Design review of the part built by this model. Coordinates are the model's own, in mm. Face numbers are marked on the shaded views. A direction names the side the tool comes from. Give positions to 0.01 mm unless a question says otherwise; leave off trailing zeros. Write each loop counter-clockwise with the first axis right and the second up, starting at its lowest first coordinate (ties: lowest second). Pieces come first, ordered by that corner, then holes. Notation, with made-up numbers: (21, 75.25) -> (59, 75.25) arc R17 ccw to (59, 97.25) -> close; hole circle Ø1 at (67.5, 54.5). An arc over 180 degrees is marked (long way). Write each question's results on one line, items separated by ' | '. Start each with the question number.
(1) Take a section at A-A (z = 0). State the section outline as (x, y) points, plus the area to 3 significant figures.
(2) Take a section at C-C (z = 27). State the section outline as (x, y) points.
(3) Clearance check with flat-ended pins moving along their axes: pin 1 (1.6 mm diameter, centred on x = -2.5, y = 9, fed in from +Z); pin 2 (12 mm diameter, centred on y = 16.5, z = 14, fed in from +X); pin 3 (2 mm diameter, centred on x = 18, y = 5, fed in from +Z). State where each tip first meets the part, or that it passes through.
(4) Take a section at B-B (y = 17.75). State the section outline as (x, z) points, plus the area to 3 significant figures.
(5) Mouldability with a two-part tool opening along X and no side actions: class the marked faces 1, 2 and 3 as released by +X, released by -X, zero draft, split by the parting line, or undercut.
(6) Take a section at D-D (z = 17). State the section outline as (x, y) points, plus the area to 3 significant figures.
(7) To check wall thickness, follow probe 1 along Y at (x, z) = (20, 4); probe 2 along X at (y, z) = (14.5, 1); probe 3 along Z at (x, y) = (0.5, 3.75). State the ranges of each line that lie inside material, in increasing order.
(8) For the marked faces 4, 5 and 6, list the 3-axis set-ups (+Z, -Z, +X, -X, +Y, -Y) from which the entire face can be reached by the end or side of a thin tool; tool diameter is ignored.
from build123d import *

# Parameters (mm, degrees)
SALIENTE_EXTRUIR1_DEPTH    = 20
CROQUIS2_R                 = 3.5
CORTAR_EXTRUIR1_DEPTH      = 34.346664001
CORTAR_EXTRUIR2_DEPTH      = 34.346664001
CORTAR_EXTRUIR2_DEPTH_BACK = 34.346664001
CROQUIS3_R                 = 1.5
CROQUIS4_R                 = 3.25
CORTAR_EXTRUIR3_DEPTH      = 1
SALIENTE_EXTRUIR2_DEPTH    = 20
CORTAR_EXTRUIR4_DEPTH      = 53.117655446
CORTAR_EXTRUIR4_DEPTH_BACK = 53.117655446
CROQUIS7_R                 = 1.75
CORTAR_EXTRUIR5_DEPTH      = 2
REDONDEO1_R                = 1


with BuildPart() as part:
    # Croquis1 → Saliente-Extruir1 (new body)
    with BuildSketch(Plane(origin=(0, 0, 0), x_dir=(1, 0, 0), z_dir=(0, 1, 0))):
        with BuildLine():
            Line((-20, 6), (20, 6))
            ThreePointArc((20, 6), (26, 0), (20, -6))
            Line((20, -6), (-20, -6))
            ThreePointArc((-20, -6), (-26, 0), (-20, 6))
        make_face()
    extrude(amount=SALIENTE_EXTRUIR1_DEPTH)

    # Croquis2 → Cortar-Extruir1 (cut, through all)
    with BuildSketch(Plane(origin=(0, 0, 0), x_dir=(1, 0, 0), z_dir=(0, 1, 0))):
        with Locations(Location((-20, 0, 0), (0, 0, 270))):
            Circle(CROQUIS2_R)
        with Locations(Location((20, 0, 0), (0, 0, 270))):
            Circle(CROQUIS2_R)
    extrude(amount=CORTAR_EXTRUIR1_DEPTH, mode=Mode.SUBTRACT)

    # Croquis3 → Cortar-Extruir2 (cut, two sides: drawn at the far end of the back side and taken through both)
    with BuildSketch(Plane.XY.offset(-CORTAR_EXTRUIR2_DEPTH_BACK)):
        with Locations(Location((-20, 10, 0), (0, 0, 270))):
            Circle(CROQUIS3_R)
        with Locations(Location((20, 10, 0), (0, 0, 270))):
            Circle(CROQUIS3_R)
    extrude(amount=CORTAR_EXTRUIR2_DEPTH + CORTAR_EXTRUIR2_DEPTH_BACK, mode=Mode.SUBTRACT)

    # Croquis4 → Cortar-Extruir3 (cut)
    with BuildSketch(Plane.XY.offset(6)):
        with Locations((-20, 10)):
            Circle(CROQUIS4_R)
        with Locations(Location((20, 10, 0), (0, 0, 270.000000001))):
            Circle(CROQUIS4_R)
    extrude(amount=-CORTAR_EXTRUIR3_DEPTH, mode=Mode.SUBTRACT)

    # Croquis6 → Saliente-Extruir2 (add)
    with BuildSketch(Plane.XZ):
        with BuildLine():
            Line((-4, 6), (-4, 16.157280718))
            ThreePointArc((-4, 16.157280718), (0, 40.5), (4, 16.157280718))
            Line((4, 16.157280718), (4, 7))
            Line((4, 7), (1, 7))
            Line((1, 7), (1, 19.559028492))
            ThreePointArc((1, 19.559028492), (-0.500870333, 36.485230045), (0, 19.5))
            Line((0, 19.5), (0, 6))
            Line((0, 6), (-4, 6))
        make_face()
    extrude(amount=-SALIENTE_EXTRUIR2_DEPTH)

    # Croquis7 → Cortar-Extruir4 (cut, two sides: drawn at the far end of the back side and taken through both)
    with BuildSketch(Plane(origin=(0, 0, 0), x_dir=(0, 0, -1), z_dir=(1, 0, 0)).offset(-CORTAR_EXTRUIR4_DEPTH_BACK)):
        with Locations((-11.578640359, 10)):
            Circle(CROQUIS7_R)
    extrude(amount=CORTAR_EXTRUIR4_DEPTH + CORTAR_EXTRUIR4_DEPTH_BACK, mode=Mode.SUBTRACT)

    # Croquis8 → Cortar-Extruir5 (cut)
    with BuildSketch(Plane.ZY.offset(4)):
        Polygon((11.578640359, 13.75277675), (8.328640359, 11.876388375), (8.328640359, 8.123611625), (11.578640359, 6.24722325), (14.828640359, 8.123611625), (14.828640359, 11.876388375), align=None)
    extrude(amount=-CORTAR_EXTRUIR5_DEPTH, mode=Mode.SUBTRACT)

    # Redondeo1
    redondeo1_edges = [part.edges().sort_by_distance(p)[0] for p in [
        (0, 10, 19.5),
        (-4, 10, 6),
        (-4, 10, 16.157280718),
        (4, 10, 16.157280718),
        (4, 10, 7),
        (1, 10, 7),
        (1, 10, 19.559028492),
        (2.5, 0, 7),
        (2.5, 20, 7),
    ]]
    fillet(redondeo1_edges, radius=REDONDEO1_R)


solid = part.part
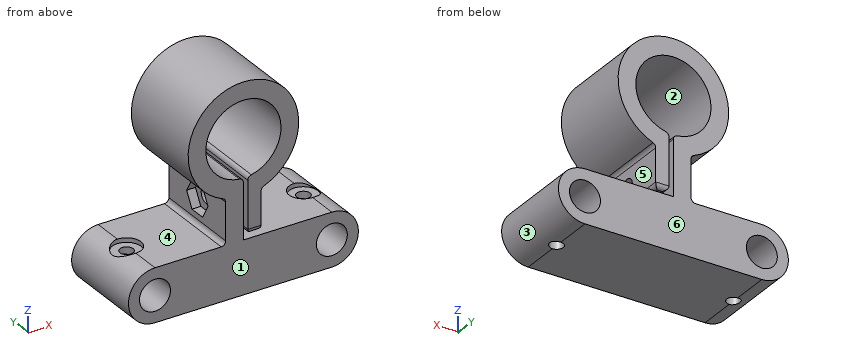
Report:
1) outline: (-26, 0) -> (-23.5, 0) -> (-23.5, 20) -> (-26, 20) -> close; (-16.5, 0) -> (16.5, 0) -> (16.5, 20) -> (-16.5, 20) -> close; (23.5, 0) -> (26, 0) -> (26, 20) -> (23.5, 20) -> close | area: 760 mm2
2) outline: (-12.46, 0) -> (-8.44, 0) -> (-8.44, 20) -> (-12.46, 20) -> close; (8.44, 0) -> (12.46, 0) -> (12.46, 20) -> (8.44, 20) -> close
3) pin 1: z = 40.38 | pin 2: x = 9.6 | pin 3: z = 6
4) outline: (-20, -6) -> (20, -6) arc R6 ccw to (20, 6) -> (0, 6) -> (0, 18.55) arc R1 ccw to (-0.89, 19.55) arc R8.5 cw (long way) to (1.79, 19.69) arc R1 ccw to (1, 18.71) -> (1, 8) arc R1 ccw to (2, 7) -> (3, 7) arc R1 ccw to (4, 8) -> (4, 15.46) arc R1 cw to (4.63, 16.39) arc R12.5 ccw (long way) to (-4.63, 16.39) arc R1 cw to (-4, 15.46) -> (-4, 7) arc R1 cw to (-5, 6) -> (-20, 6) arc R6 ccw to start; hole circle Ø7 at (-20, 0); hole circle Ø7 at (20, 0) | area: 841 mm2
5) face 1: zero draft | face 2: undercut | face 3: released by +X
6) outline: (-5.94, 0) -> (0, 0) -> (0, 20) -> (-5.94, 20) -> close; (1, 0) -> (5.94, 0) -> (5.94, 20) -> (1, 20) -> close | area: 217 mm2
7) probe 1: 0 to 8.5, 11.5 to 20 | probe 2: -25.92 to -23.35, -16.65 to 16.65, 23.35 to 25.92 | probe 3: -6 to 6, 36.49 to 40.49
8) face 4: -X, +Y, -Y | face 5: +X, +Y, -Y | face 6: +Z, -Z, +X, -X, +Y
